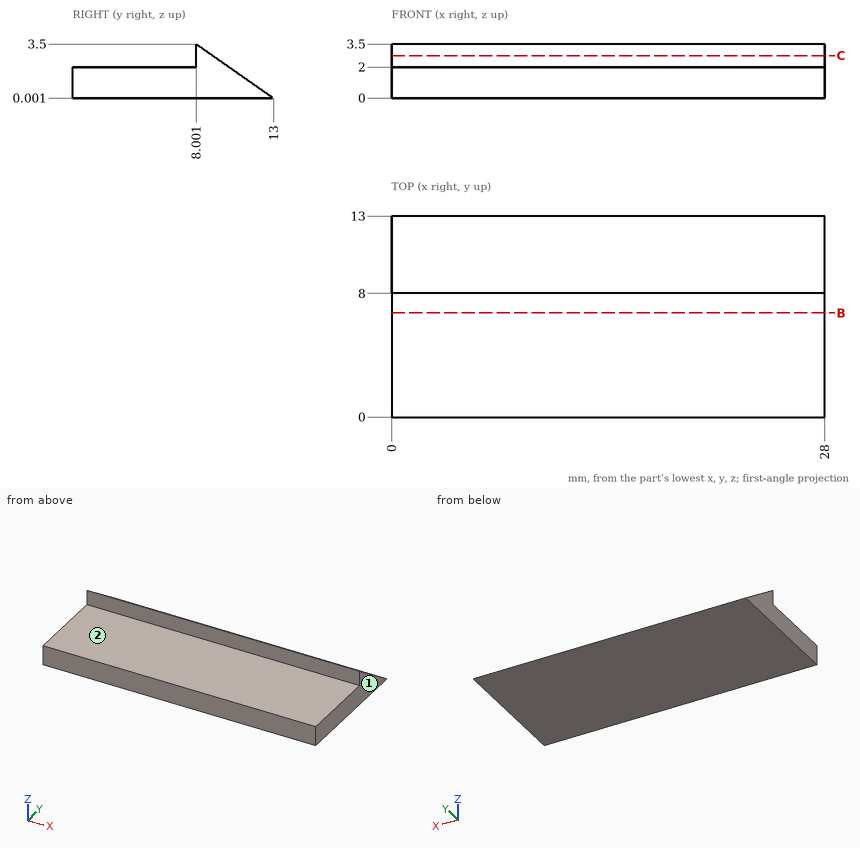
The figure shows three views and two pictorial views of one solid part (mm, origin at its lowest corner). Answer the questions. A direction names the side the tool comes from. Round coordinates to 2 decimals unless told otherwise and drop trailing zeros. Loops run counter-clockwise (first coordinate to the right, second up) from the corner with the lowest first, then second, coordinate; pieces in that order, holes last. Notation, with made-up numbers: M -25.5,5.5 L 26.5,5.5 A20 cw 26.5,29.5 Z; hole C 15.25,89.5 d6. An arc over 180 degrees is marked long. Use CSV: the item, a comma, the result in double quotes.
Q1. Section B-B, the plane y = 6.75 is taken. Determine the outline of the cut face in (x, z).
Determined:
outline,"M 0,0 L 28,0 L 28,2 L 0,2 Z"
Q2. A tool of negligible diameter and unlimited length cuts with its end or side. For the marked faces 1 and 2, from which of +Z, -Z, +X, -X, +Y, -Y can it reach the whole face along a straight path? Write none if from no direction.
Determined:
face 1,"+Z, -Z, +X, +Y, -Y"
face 2,"+Z, +X, -X, -Y"
Q3. Section C-C, the plane z = 2.75 is taken. Determine the outline of the cut face in (x, y).
Determined:
outline,"M 0,8 L 28,8 L 28,9.07 L 0,9.07 Z"
Q4. Each of these flat-tipped pins is pushed along its axis until it touches: pin 1 (1.5 mm diameter, centred on x = 23, y = 9, fed in from -Z); pin 2 (6 mm diameter, centred on x = 4.5, y = 3, fed in from +Z); pin 3 (1.6 mm diameter, centred on x = 11.5, z = 3, fed in from -Y); pin 4 (1 mm diameter, centred on x = 11.5, z = 1, fed in from +Y). Where does it stop, or does it pass through?
Determined:
pin 1,"z = 0"
pin 2,"z = 2"
pin 3,"y = 8"
pin 4,"y = 12.29"
Q5. Consider L1, parallel to Z at x = 26, y = 6.25; L2, parallel to Y at x = 2.5, z = 0.65; L3, parallel to Y at x = 21, z = 2.4. Determine where each line is inside the solid, lowest interval first.
Determined:
L1,"0 to 2"
L2,"0 to 12.07"
L3,"8 to 9.57"
